```python
from build123d import *

# Parameters (mm, degrees)
CHAMFER1_SIZE = 1


with BuildPart() as part:
    # Sketch2 → Revolve1 (revolve)
    with BuildSketch(Plane(origin=(0, 0, 0), x_dir=(0, 0, -1), z_dir=(1, 0, 0))):
        Polygon((2.5, 0), (2.5, 3.375), (4, 3.375), (4, 6.5), (7, 6.5), (7, 6), (6, 5), (6, 0), align=None)
    revolve1 = revolve(axis=Axis((0, 0, 0), (0, 1, 0)))

    # Mirror1: Revolve1 across plane
    add(revolve1.mirror(Plane.ZX))

    # Chamfer1
    chamfer1_edges = [part.edges().sort_by_distance(p)[0] for p in [
        (0, -3.375, 2.5),
        (0, 3.375, 2.5),
    ]]
    chamfer(chamfer1_edges, length=CHAMFER1_SIZE)


solid = part.part
```
The listing builds one solid part. Answer for the finished solid, in the listing's coordinates (mm). Coordinates: 2 decimals unless noted, no trailing zeros. Loops run counter-clockwise (first coordinate to the right, second up) from the corner with the lowest first, then second, coordinate; pieces in that order, holes last. Notation, with made-up numbers: (-32, 47) - (-17, 47) arc R8 cw to (-17, 59) - close; hole circle Ø6 at (45, -6.75). An arc over 180 degrees is marked (long way). Write item = value, one per line.
1) Find the intervals of material crossed by line 1 along X through (y, z) = (-1.65, 0); line 2 along X through (y, z) = (4.75, 0), in increasing order.
Responses:
line_1 = -6 to -2.5, 2.5 to 6
line_2 = -6 to -4, 4 to 6
2) Section D-D (y = 5.25) is taken. Determine the outline of the cut face in (x, z).
Responses:
outline = circle Ø12.5 at (0, 0); hole circle Ø8 at (0, 0)
3) Section C-C (y = -1.5) is taken. Determine the outline of the cut face in (x, z), plus the area to 3 significant figures.
Responses:
outline = circle Ø12 at (0, 0); hole circle Ø5 at (0, 0)
area = 93.5 mm^2
4) Section B-B (z = 0) is taken. Determine the outline of the cut face in (x, y) (3 decimals).
Responses:
outline = (-7, -6.5) - (-4, -6.5) - (-4, -3.375) - (-3.5, -3.375) - (-2.5, -2.375) - (-2.5, 2.375) - (-3.5, 3.375) - (-4, 3.375) - (-4, 6.5) - (-7, 6.5) - (-7, 6) - (-6, 5) - (-6, -5) - (-7, -6) - close; (2.5, -2.375) - (3.5, -3.375) - (4, -3.375) - (4, -6.5) - (7, -6.5) - (7, -6) - (6, -5) - (6, 5) - (7, 6) - (7, 6.5) - (4, 6.5) - (4, 3.375) - (3.5, 3.375) - (2.5, 2.375) - close
5) Each of these flat-tipped pins is pushed along its axis until it touches: P1, Ø1, axis at y = 4, z = 2, coming from the +X side; P2, Ø6.5, axis at x = 0, z = 0, coming from the +Y side (3 decimals); P3, Ø1, axis at y = -2, z = -3, coming from the -X side. Where does it stop, or does it pass through?
Responses:
P1 = 5.81
P2 = 3.125
P3 = -5.45
6) Determine the mould class of faces 1 (the face through (2.681, -6.246, -6.466)), 2 (the face through (3, 6.5, 3)), 3 (the face through (3.905, -4.959, 0.867)), 4 (the face through (3.905, 4.959, 0.867)) for opening direction Z: pulls with the +Z half, pulls with the -Z half, needs draft (parallel to the pull), parting line crosses it, or undercut.
Responses:
face_1 = parting line crosses it
face_2 = needs draft
face_3 = undercut
face_4 = undercut
7) Section A-A (x = 0) is taken. Determine the outline of the cut face in (y, z) (3 decimals).
Responses:
outline = (-6.5, -7) - (-6, -7) - (-5, -6) - (5, -6) - (6, -7) - (6.5, -7) - (6.5, -4) - (3.375, -4) - (3.375, -3.5) - (2.375, -2.5) - (-2.375, -2.5) - (-3.375, -3.5) - (-3.375, -4) - (-6.5, -4) - close; (-6.5, 4) - (-3.375, 4) - (-3.375, 3.5) - (-2.375, 2.5) - (2.375, 2.5) - (3.375, 3.5) - (3.375, 4) - (6.5, 4) - (6.5, 7) - (6, 7) - (5, 6) - (-5, 6) - (-6, 7) - (-6.5, 7) - close
